Work out the finished part from the listing and answer in its coordinate system (mm). Face numbers are marked on the shaded views. A direction names the side the tool comes from. Round coordinates to 2 decimals unless told otherwise and drop trailing zeros. Order: outer loops, then holes, each group sorted by start corner. A loop starts at its lowest first (then second) coordinate and runs counter-clockwise, first axis right, second up. Notation, with made-up numbers: (36, -37.75) -> (67, -37.75) arc R11 cw to (67, -19.75) -> close; hole circle Ø5 at (38, 50.5). An arc over 180 degrees is marked (long way). Use a Markdown table: item, result. Add a question column.
Item 1: Flat-ended cylindrical pins translate along their axes: P1, Ø9.5, axis at x = 31.5, z = 3, coming from the +Y side; P2, Ø1.8, axis at x = -40.9, z = -3.25, coming from the +Y side; P3, Ø10, axis at y = 11.5, z = -2, coming from the -X side. Find the tip coordinate at first contact, or state that the pin passes through.
Item 2: A cutting plane is placed at B-B, the plane y = -1. Give the number of separate pieces and of enclosed holes in the cut face, plus the area to 3 significant figures.
Item 3: For a pull along X with two mould halves and no side action, classify the marked faces 6, 7 and 8 as +X half, -X half, draft (parallel to the pull), parting line (faces both ways), or undercut.
Item 4: A tool of negligible diameter and unlimited length cuts with its end or side. For the marked faces 1, 2, 3, 4 and 5, from which of +Z, -Z, +X, -X, +Y, -Y can it reach the whole face along a straight path? Write none if from no direction.
Item 5: Find the intervals of material crossed by L1, parallel to Z at x = -40.9, y = -4.25; L2, parallel to X at y = -2.25, z = -3.25; L3, parallel to X at y = -1.25, z = -3.25, in increasing order. Write a range as [from, to].
Item 6: A cutting plane is placed at A-A, the plane x = -16.5. Determine the outline of the cut face in (y, z).
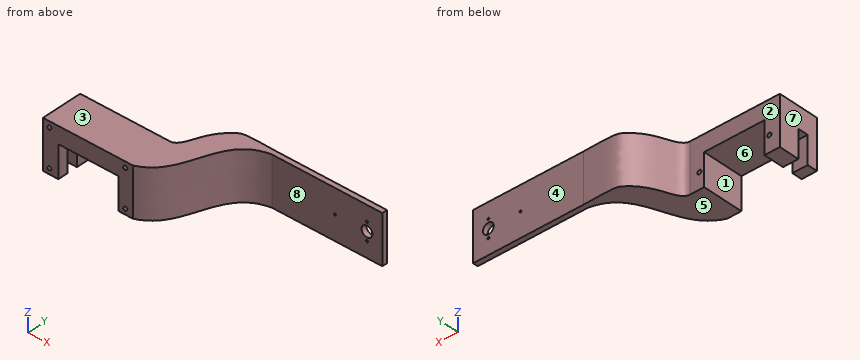
from build123d import *

# Parameters (mm, degrees)
SKETCH1_W            = 35
SKETCH1_H            = 19
BOSS_EXTRUDE1_DEPTH  = 2
SKETCH2_W            = 35
SKETCH2_H            = 19
BOSS_EXTRUDE2_DEPTH  = 14
SKETCH5_W            = 23.5
SKETCH5_H            = 12.5
CUT_EXTRUDE1_DEPTH   = 16
SKETCH6_W            = 12
SKETCH6_H            = 4
CUT_EXTRUDE2_DEPTH   = 35
BOSS_EXTRUDE7_DEPTH  = 19
SKETCH17_W           = 19
SKETCH17_H           = 2
BOSS_EXTRUDE8_DEPTH  = 40
SKETCH10_R           = 0.713910761
BOSS_EXTRUDE9_DEPTH  = 0.5
FILLET2_R            = 0.5
SKETCH18_R           = 0.4
CUT_EXTRUDE6_DEPTH   = 10.5
SKETCH19_R           = 2.1
CUT_EXTRUDE7_DEPTH   = 10.5
SKETCH20_W           = 19
SKETCH20_H           = 2
BOSS_EXTRUDE10_DEPTH = 3
SKETCH7_R            = 0.8
CUT_EXTRUDE8_DEPTH   = 8


with BuildPart() as part:
    # Sketch1 → Boss-Extrude1 (new body)
    with BuildSketch(Plane(origin=(0, 0, 0), x_dir=(1, 0, 0), z_dir=(0, 1, 0))):
        with Locations((-27.5, 0)):
            Rectangle(SKETCH1_W, SKETCH1_H)
    extrude(amount=BOSS_EXTRUDE1_DEPTH)

    # Sketch2 → Boss-Extrude2 (add)
    with BuildSketch(Plane(origin=(0, 0, 0), x_dir=(-1, 0, 0), z_dir=(0, -1, 0))):
        with Locations((27.5, 0)):
            Rectangle(SKETCH2_W, SKETCH2_H)
    extrude(amount=BOSS_EXTRUDE2_DEPTH)

    # Sketch5 → Cut-Extrude1 (cut)
    with BuildSketch(Plane(origin=(0, 2, 0), x_dir=(1, 0, 0), z_dir=(0, 1, 0))):
        with Locations((-27.25, 3.25)):
            Rectangle(SKETCH5_W, SKETCH5_H)
    extrude(amount=-CUT_EXTRUDE1_DEPTH, mode=Mode.SUBTRACT)

    # Sketch6 → Cut-Extrude2 (cut)
    with BuildSketch(Plane.ZY.offset(15.5)):
        with Locations((-4.723551551, -8)):
            Rectangle(SKETCH6_W, SKETCH6_H)
    extrude(amount=CUT_EXTRUDE2_DEPTH, mode=Mode.SUBTRACT)

    # Sketch15 → Boss-Extrude7 (add)
    with BuildSketch(Plane.XY.offset(9.5)):
        with BuildLine():
            Line((16.244255375, 17), (16.244255375, 19))
            add(Edge.make_bspline(
                [(16.244255375, 19), (11.212607589, 19), (4.066469068, 19.553217376), (-0.106803104, 16.983328742), (-5.242294622, 11.037813369), (-6.977758039, 2), (-10, 2)],
                knots=[0, 0, 0, 0, 0.246137696, 0.311425048, 0.652873521, 1, 1, 1, 1], degree=3))
            Line((-10, 2), (-10, -14))
            add(Edge.make_bspline(
                [(-10, -14), (5.215691354, -8.082881299), (-1.571658903, 13.967697147), (16.244255375, 17)],
                knots=[0, 0, 0, 0, 1, 1, 1, 1], degree=3))
        make_face()
    extrude(amount=-BOSS_EXTRUDE7_DEPTH)

    # Sketch17 → Boss-Extrude8 (add)
    with BuildSketch(Plane(origin=(16.244255375, 0, 0), x_dir=(0, 0, -1), z_dir=(1, 0, 0))):
        with Locations((0, 18)):
            Rectangle(SKETCH17_W, SKETCH17_H)
    extrude(amount=BOSS_EXTRUDE8_DEPTH)

    # Sketch10 → Boss-Extrude9 (add)
    with BuildSketch(Plane(origin=(0, -14, 0), x_dir=(-1, 0, 0), z_dir=(0, -1, 0))):
        with Locations(Location((42.426696663, 7.292088489, 0), (0, 0, 90))):
            Circle(SKETCH10_R)
        with Locations(Location((12.850393701, 7.292088489, 0), (0, 0, 90))):
            Circle(SKETCH10_R)
        with Locations(Location((12.850393701, -7.292088489, 0), (0, 0, 270))):
            Circle(SKETCH10_R)
        with Locations(Location((42.426696663, -7.292088489, 0), (0, 0, 270))):
            Circle(SKETCH10_R)
    extrude(amount=BOSS_EXTRUDE9_DEPTH)

    # Fillet2
    fillet2_edges = [part.edges().sort_by_distance(p)[0] for p in [
        (-12.850393701, -14.5, 6.578177728),
        (-42.426696663, -14.5, 6.578177728),
        (-42.426696663, -14.5, -6.578177728),
        (-12.850393701, -14.5, -6.578177728),
    ]]
    fillet(fillet2_edges, radius=FILLET2_R - 0.0001)  # a hair under: the kernel refuses the full size

    # Sketch18 → Cut-Extrude6 (cut)
    with BuildSketch(Plane(origin=(0, 19, 0), x_dir=(1, 0, 0), z_dir=(0, 1, 0))):
        with Locations(Location((53.244255375, 3.45, 0), (0, 0, 270))):
            Circle(SKETCH18_R)
        with Locations(Location((53.244255375, -3.45, 0), (0, 0, 270))):
            Circle(SKETCH18_R)
        with Locations((50.214832051, 25.851748831)):
            Circle(SKETCH18_R)
        with Locations(Location((40.744255375, 0, 0), (0, 0, 270))):
            Circle(SKETCH18_R)
    extrude(amount=-CUT_EXTRUDE6_DEPTH, mode=Mode.SUBTRACT)

    # Sketch19 → Cut-Extrude7 (cut)
    with BuildSketch(Plane(origin=(0, 19, 0), x_dir=(1, 0, 0), z_dir=(0, 1, 0))):
        with Locations(Location((53.244255375, 0, 0), (0, 0, 270))):
            Circle(SKETCH19_R)
    extrude(amount=-CUT_EXTRUDE7_DEPTH, mode=Mode.SUBTRACT)

    # Sketch20 → Boss-Extrude10 (add)
    with BuildSketch(Plane(origin=(56.244255375, 0, 0), x_dir=(0, 0, -1), z_dir=(1, 0, 0))):
        with Locations((0, 18)):
            Rectangle(SKETCH20_W, SKETCH20_H)
    extrude(amount=BOSS_EXTRUDE10_DEPTH)

    # Sketch7 → Cut-Extrude8 (cut)
    with BuildSketch(Plane(origin=(0, 2, 0), x_dir=(1, 0, 0), z_dir=(0, 1, 0))):
        with Locations(Location((-40.9, 3.25, 0), (0, 0, 270))):
            Circle(SKETCH7_R)
        with Locations(Location((-13.6, 3.25, 0), (0, 0, 270))):
            Circle(SKETCH7_R)
    extrude(amount=-CUT_EXTRUDE8_DEPTH, mode=Mode.SUBTRACT)


solid = part.part
Reported:
| question | item | result |
|---|---|---|
| 1 | P1 | y = 19 |
| 1 | P2 | y = 2 |
| 1 | P3 | x = -5.94 |
| 2 | separate pieces | 1 |
| 2 | enclosed holes | 2 |
| 2 | area | 573 mm² |
| 3 | face 6 | undercut |
| 3 | face 7 | -X half |
| 3 | face 8 | draft |
| 4 | face 1 | -Z, +Y, -Y |
| 4 | face 2 | +Z, -Z, -X, +Y |
| 4 | face 3 | +Z, +X, -X, +Y, -Y |
| 4 | face 4 | +Z, -Z, +X, +Y |
| 4 | face 5 | -Z, +X, -X, +Y, -Y |
| 5 | L1 | [-9.5, -4.05], [-2.45, 9.5] |
| 5 | L2 | [-45, -41.7], [-40.1, -39], [-15.5, -14.4], [-12.8, 0.35] |
| 5 | L3 | [-45, -41.7], [-40.1, -39], [-15.5, -14.4], [-12.8, 0.74] |
| 6 | outline | (-14, 3) -> (2, 3) -> (2, 9.5) -> (-14, 9.5) -> close |
